Check sheet for the modelled part. Datum: model origin and axes. Units: mm. Coordinates: 2 decimals unless noted, no trailing zeros. Loops run counter-clockwise (first coordinate to the right, second up) from the corner with the lowest first, then second, coordinate; pieces in that order, holes last. Notation, with made-up numbers: M 88,41 L 116,41 A18 cw 116,60 Z; hole C 88,-17.75 d1. An arc over 180 degrees is marked long. Return JSON: item names as keys, results as strings.
from build123d import *

# Parameters (mm, degrees)
SKETCH1_W                = 50
SKETCH1_H                = 16
BOSS_EXTRUDE1_DEPTH      = 3
BOSS_EXTRUDE1_DEPTH_BACK = 3


with BuildPart() as part:
    # Sketch1 → Boss-Extrude1 (new body, two sides)
    with BuildSketch(Plane.XY) as boss_extrude1_sk:
        with Locations((15, 0)):
            Rectangle(SKETCH1_W, SKETCH1_H)
    extrude(amount=BOSS_EXTRUDE1_DEPTH)
    extrude(boss_extrude1_sk.sketch, amount=-BOSS_EXTRUDE1_DEPTH_BACK)

    # Sketch2 → Cut-Revolve1 (revolve, cut)
    with BuildSketch(Plane(origin=(0, 0, 0), x_dir=(0, 0, -1), z_dir=(1, 0, 0))):
        Polygon((-3, 0), (-3, 3), (-2.4585, 2.4585), (2.4585, 2.4585), (3, 3), (3, 0), align=None)
    revolve(axis=Axis((0, 0, -3), (0, 0, 1)), mode=Mode.SUBTRACT)

    # Sketch3 → Cut-Revolve2 (revolve, cut)
    with BuildSketch(Plane(origin=(30, 0, 0), x_dir=(0, 0, -1), z_dir=(1, 0, 0))):
        Polygon((-3, 0), (-3, 3), (-2.4585, 2.4585), (2.4585, 2.4585), (3, 3), (3, 0), align=None)
    revolve(axis=Axis((30, 0, -3), (0, 0, 1)), mode=Mode.SUBTRACT)


solid = part.part
1) Section check C-C on z = -0.65. Record the cut outline in (x, y).
Answers:
{"outline": "M -10,-8 L 40,-8 L 40,8 L -10,8 Z; hole C 0,0 d4.92; hole C 30,0 d4.92"}
2) Section check A-A on y = 0. Record the cut outline in (x, z), then the cut area to 3 significant figures.
Answers:
{"outline": "M -10,-3 L -3,-3 L -2.46,-2.46 L -2.46,2.46 L -3,3 L -10,3 Z; M 2.46,-2.46 L 3,-3 L 27,-3 L 27.54,-2.46 L 27.54,2.46 L 27,3 L 3,3 L 2.46,2.46 Z; M 32.46,-2.46 L 33,-3 L 40,-3 L 40,3 L 33,3 L 32.46,2.46 Z", "area": "240 mm²"}
3) Scan lines: line 1 along X through (y, z) = (0, -0.6); line 2 along X through (y, z) = (-2.25, 1.15); line 3 along Y through (x, z) = (0, -0.45). Record each from-to range of solid material in increasing order. Write a range as [from, to].
Answers:
{"line 1": "[-10, -2.46], [2.46, 27.54], [32.46, 40]", "line 2": "[-10, -0.99], [0.99, 29.01], [30.99, 40]", "line 3": "[-8, -2.46], [2.46, 8]"}
4) Section check D-D on y = -2. Count the separate pieces of the cut face and the enclosed holes in it, then the cut area to 3 significant figures.
Answers:
{"separate pieces": "3", "enclosed holes": "0", "area": "264 mm²"}
5) Section check B-B on x = 0. Record the cut outline in (y, z), then the cut area to 3 significant figures.
Answers:
{"outline": "M -8,-3 L -3,-3 L -2.46,-2.46 L -2.46,2.46 L -3,3 L -8,3 Z; M 2.46,-2.46 L 3,-3 L 8,-3 L 8,3 L 3,3 L 2.46,2.46 Z", "area": "65.9 mm²"}
6) Go/stop test with flat-tipped pins: pin 1 Ø4.5 at (x, y) = (30, 0) entering from -Z; pin 2 Ø5.5 at (x, y) = (0, 0) entering from -Z. Record where each tip stops, or that it passes through.
Answers:
{"pin 1": "through", "pin 2": "z = -2.75"}
